Design review of the part built by this model. Coordinates are the model's own, in mm. A direction names the side the tool comes from. Round coordinates to 2 decimals unless told otherwise and drop trailing zeros. Order: outer loops, then holes, each group sorted by start corner. A loop starts at its lowest first (then second) coordinate and runs counter-clockwise, first axis right, second up. Notation, with made-up numbers: M 74.25,76 L 81.25,76 A30 cw 81.25,109 Z; hole C 69,-21 d10. An arc over 180 degrees is marked long. Use a Markdown table: item, result. Add a question column.
(1) Take a section at B-B (x = 16.5). Write out the cut boundary in (y, z), then the cut area to 3 significant figures.
(2) Machinability: for faces 1 (the face through (37.134, -6, -1)), 2 (the face through (19, 0, 0)), which of the approach directions +Z, -Z, +X, -X, +Y, -Y give a long, thin tool a straight path to every point of the face, cutting with its end or side? Answer none if there is none.
(3) Take a section at A-A (z = -6.5). Write out the cut boundary in (x, y), then the cut area to 3 significant figures.
(4) To check wall thickness, follow probe 1 along Y at (x, z) = (16, -3.75); probe 2 along Y at (x, z) = (24.75, -0.75). State the ranges of each line that lie inside material, in increasing order. Write a range as from..to.
(5) For pin 1 (2 mm diameter, centred on x = 34, z = -6.5, fed in from +Y); pin 2 (1.5 mm diameter, centred on y = 2.5, z = -1.5, fed in from -X); pin 3 (7.5 mm diameter, centred on x = 19.5, z = -2.5, fed in from +Y), all flat-tipped, find the tip position at first contact; note any pin that passes through.
```python
from build123d import *

# Parameters (mm, degrees)
F0_W     = 25.4
F0_H     = 25.4
F1_DEPTH = 12.7
F2_R     = 5.08
F3_DEPTH = 5.08
F4_R     = 5.07999


# Not quite as in the source:
# - a fillet or chamfer is up to 0.001 mm smaller than in the source, because OpenCascade refuses the exact size


with BuildPart() as f1:
    # F0 (on Front) → F1 (new body)
    with BuildSketch(Plane.XZ):
        with Locations((24.4342711151, -0.3571881309)):
            Rectangle(F0_W, F0_H)
    extrude(amount=F1_DEPTH)

    # F2 (on Front) → F3 (join)
    with BuildSketch(Plane.XZ):
        with Locations((24.4607284337, 0)):
            Circle(F2_R)
    extrude(amount=-F3_DEPTH)

    # F4 (radius 5.08 in the source; OpenCascade refuses exactly that, so slightly less here)
    f4_edges = [f1.edges().sort_by_distance(p)[0] for p in [
        (19.380728, 5.08, 0),
    ]]
    fillet(f4_edges, radius=F4_R)


solid = f1.part
```
Verdict:
| question | item | result |
|---|---|---|
| 1 | outline | M -12.7,-13.06 L 0,-13.06 L 0,12.34 L -12.7,12.34 Z |
| 1 | area | 323 mm^2 |
| 2 | face 1 | +Z, -Z, +X, +Y, -Y |
| 2 | face 2 | +Y |
| 3 | outline | M 11.73,-12.7 L 37.13,-12.7 L 37.13,0 L 11.73,0 Z |
| 3 | area | 323 mm^2 |
| 4 | probe 1 | y = -12.7..0 |
| 4 | probe 2 | y = -12.7..5.02 |
| 5 | pin 1 | stops at y = 0 |
| 5 | pin 2 | stops at x = 19.87 |
| 5 | pin 3 | stops at y = 4.75 |
